Verification items for the finished model (mm, model axes). A direction names the side the tool comes from. Give positions to 0.01 mm unless a question says otherwise; leave off trailing zeros. Order: outer loops, then holes, each group sorted by start corner. A loop starts at its lowest first (then second) coordinate and runs counter-clockwise, first axis right, second up.
from build123d import *

# Parameters (mm, degrees)
SKETCH1_R           = 3.175
BOSS_EXTRUDE1_DEPTH = 3.175
SKETCH3_R           = 3.175
BOSS_EXTRUDE2_DEPTH = 3.175
SKETCH4_R           = 6.35
SKETCH4_R_2         = 3.175
BOSS_EXTRUDE3_DEPTH = 6.35
FILLET1_R           = 6.35


with BuildPart() as part:
    # Sketch1 → Boss-Extrude1 (new body)
    with BuildSketch(Plane(origin=(0, 0, 0), x_dir=(0, 0, -1), z_dir=(1, 0, 0))):
        with BuildLine():
            ThreePointArc((3.174007657, -63.420625), (0, -60.325), (-3.174007657, -63.420625))
            ThreePointArc((-3.174007657, -63.420625), (0, 63.5), (3.174007657, -63.420625))
        make_face()
        Circle(SKETCH1_R, mode=Mode.SUBTRACT)
    extrude(amount=BOSS_EXTRUDE1_DEPTH)

    # Sketch3 → Boss-Extrude2 (add)
    with BuildSketch(Plane(origin=(3.175, 0, 0), x_dir=(0, 0, -1), z_dir=(1, 0, 0))):
        Polygon((0, 21.997045256), (-19.05, -10.998522628), (19.05, -10.998522628), align=None)
        Circle(SKETCH3_R, mode=Mode.SUBTRACT)
    extrude(amount=BOSS_EXTRUDE2_DEPTH)

    # Sketch4 → Boss-Extrude3 (add)
    with BuildSketch(Plane(origin=(6.35, 0, 0), x_dir=(0, 0, -1), z_dir=(1, 0, 0))):
        Circle(SKETCH4_R)
        Circle(SKETCH4_R_2, mode=Mode.SUBTRACT)
    extrude(amount=BOSS_EXTRUDE3_DEPTH)

    # Fillet1
    fillet1_edges = [part.edges().sort_by_distance(p)[0] for p in [
        (4.7625, -10.998522628, -19.05),
        (4.7625, 21.997045256, 0),
        (4.7625, -10.998522628, 19.05),
    ]]
    fillet(fillet1_edges, radius=FILLET1_R)


solid = part.part
(1) Section check B-B, the plane z = 0. Enter the section's corners in (x, y) (3 decimals), then the cut area to 3 significant figures.
Solved:
outline: (0, -60.325) - (3.175, -60.325) - (3.175, -10.999) - (6.35, -10.999) - (6.35, -6.35) - (12.7, -6.35) - (12.7, -3.175) - (0, -3.175) - close; (0, 3.175) - (12.7, 3.175) - (12.7, 6.35) - (6.35, 6.35) - (6.35, 15.647) - (3.175, 15.647) - (3.175, 63.5) - (0, 63.5) - close
area: 478 mm2
(2) Set-up check for faces 1 (the cylindrical face through (4.78, -7.74, 13.6)), 2 (the flat face through (3.175, -13, -1)), 3 (the cylindrical face through (4.785, 15.646, 0.093)), 4 (the cylindrical face through (4.785, -7.904, -13.504)), 5 (the flat face through (4.74, 5.4, -9.58)): record each of +Z, -Z, +X, -X, +Y, -Y from which the full face is reachable in a straight line by a thin tool's end or side.
Solved:
face 1: +Z, +X
face 2: +X
face 3: +X, +Y
face 4: -Z, +X
face 5: -Z, +X, +Y
(3) Section check D-D, the plane y = -34. Enter the section's corners in (x, z) (3 decimals), then the cut area to 3 significant figures.
Solved:
outline: (0, -53.631) - (3.175, -53.631) - (3.175, 53.631) - (0, 53.631) - close
area: 341 mm2
(4) Section check A-A, the plane y = 0. Enter the section's corners in (x, z) (3 decimals).
Solved:
outline: (0, -63.5) - (3.175, -63.5) - (3.175, -12.7) - (6.35, -12.7) - (6.35, -6.35) - (12.7, -6.35) - (12.7, -3.175) - (0, -3.175) - close; (0, 3.175) - (12.7, 3.175) - (12.7, 6.35) - (6.35, 6.35) - (6.35, 12.7) - (3.175, 12.7) - (3.175, 63.5) - (0, 63.5) - close
(5) Section check C-C, the plane x = 8.5. Enter the section's corners in (y, z) (3 decimals), then the cut area to 3 significant figures.
Solved:
outline: circle Ø12.7 at (0, 0); hole circle Ø6.35 at (0, 0)
area: 95.0 mm2
(6) Scan lines: line 1 (Y direction, x = 8.5, z = 0) (3 decimals); line 2 (X direction, y = 1, z = -40.5) (3 decimals); line 3 (X direction, y = 10, z = 0). Record each from-to range of solid material in increasing order.
Solved:
line 1: y = -6.35 to -3.175, 3.175 to 6.35
line 2: x = 0 to 3.175
line 3: x = 0 to 6.35
(7) Go/stop test with flat-tipped pins: pin 1 (2.5 mm diameter, centred on x = 5, z = -0.5, fed in from -Y); pin 2 (1 mm diameter, centred on y = 25.5, z = -31, fed in from +X) (3 decimals); pin 3 (2 mm diameter, centred on x = 3, y = -45, fed in from +Z). Record where each tip stops, or that it passes through.
Solved:
pin 1: stops at y = -11
pin 2: stops at x = 3.175
pin 3: stops at z = 45.78
(8) Release check for a two-part mould opening along Y. For faces 6 (the flat face through (6.35, 3, -6)), 7 (the cylindrical face through (9.48, -6.2, 1.38)), 8 (the flat face through (5, -10.999, 0)), 9 (the cylindrical face through (6.26, -3.1, 0.69)) record: pulls with the +Y half, pulls with the -Y half, needs draft (parallel to the pull), parting line crosses it, or undercut.
Solved:
face 6: needs draft
face 7: parting line crosses it
face 8: pulls with the -Y half
face 9: undercut
